Check sheet for the modelled part. Datum: model origin and axes. Units: mm. A direction names the side the tool comes from. Coordinates: 2 decimals unless noted, no trailing zeros. Order: outer loops, then holes, each group sorted by start corner. A loop starts at its lowest first (then second) coordinate and runs counter-clockwise, first axis right, second up.
1. Cross-section at B-B (y = 0). Enter the section's corners in (x, z), then the cut area to 3 significant figures.
2. Draft check along Z on faces 4 (the flat face through (0, 8, 24)), 5 (the cylindrical face through (-49.3, 23.846, 7.509)), 6 (the flat face through (-225, 0, 125)), 7 (the flat face through (-100, 0, 0)). Enter one of: released by +Z, released by -Z, zero draft, split by the parting line, or undercut.
3. Thickness scan on line 1 (Z direction, x = -79, y = 0); line 2 (Z direction, x = -51, y = -2). Record the ranges inside material, lowest first.
4. Set-up check for faces 1 (the cylindrical face through (-76.05, -4.88, -37.18)), 2 (the flat face through (-249, -8, 475)), 3 (the cylindrical face through (-256.62, 20.16, 277.8)): record each of +Z, -Z, +X, -X, +Y, -Y from which the full face is reachable in a straight line by a thin tool's end or side.
5. Cross-section at C-C (x = -135). Enter the section's corners in (y, z).
6. Gauge pin test, flat ends, axial feed: pin 1 Ø3 at (y, z) = (3.5, 104.5) entering from -X; pin 2 Ø8 at (x, y) = (-147.5, 16) entering from -Z; pin 3 Ø1.5 at (x, z) = (-204.5, 237) entering from -Y. Record the tip position at first contact, or that the pin passes through.
7. Cross-section at A-A (z = 142.5). Enter the section's corners in (x, y).
```python
from build123d import *

# Parameters (mm, degrees)
F0_R     = 37.5
F3_R     = 25
F4_DEPTH = 350
F5_R     = 25
F6_DEPTH = 100


with BuildPart() as f2:
    # F2: sweep along a path in F1
    with BuildLine(Plane.XZ) as f2_path:
        Line((0, 0), (-150, 0))
        ThreePointArc((-150, 0), (-203.033008589, 21.966991411), (-225, 75))
        Line((-225, 75), (-225, 475))
    # F0 (on Right) → F2 (sweep)
    with BuildSketch(Plane.YZ):
        Circle(F0_R)
    sweep(path=f2_path.line)

    # F3 (on face) → F4 (cut)
    with BuildSketch(Plane.XY.offset(475)):
        with Locations((-225, 0)):
            Circle(F3_R)
    extrude(amount=-F4_DEPTH, mode=Mode.SUBTRACT)

    # F5 (on face) → F6 (cut)
    with BuildSketch(Plane.YZ):
        Circle(F5_R)
    extrude(amount=-F6_DEPTH, mode=Mode.SUBTRACT)


solid = f2.part
```
Data:
1. outline: (-262.5, 75) arc R112.5 ccw to (-150, -37.5) - (0, -37.5) - (0, -25) - (-100, -25) - (-100, 25) - (0, 25) - (0, 37.5) - (-150, 37.5) arc R37.5 cw to (-187.5, 75) - (-187.5, 475) - (-200, 475) - (-200, 125) - (-250, 125) - (-250, 475) - (-262.5, 475) - close
1. area: 27,600 mm2
2. face 4: zero draft
2. face 5: undercut
2. face 6: released by +Z
2. face 7: undercut
3. line 1: z = -37.5 to -25, 25 to 37.5
3. line 2: z = -37.45 to -24.92, 24.92 to 37.45
4. face 1: +X
4. face 2: +Z, +X, -X, +Y, -Y
4. face 3: +Z
5. outline: circle Ø75 at (0, 0)
6. pin 1: stops at x = -262.45
6. pin 2: stops at z = -35.53
6. pin 3: stops at y = -31.88
7. outline: circle Ø75 at (-225, 0); hole circle Ø50 at (-225, 0)
